from build123d import *

# Parameters (mm, degrees)
SKETCH1_W           = 135
SKETCH1_H           = 93
SKETCH1_R           = 3
BOSS_EXTRUDE1_DEPTH = 7
BOSS_EXTRUDE2_DEPTH = 39
FILLET1_R           = 10
SKETCH3_R           = 15
BOSS_EXTRUDE3_DEPTH = 22
SKETCH5_W           = 20
SKETCH5_H           = 8
BOSS_EXTRUDE4_DEPTH = 23
SKETCH6_R           = 4
CUT_EXTRUDE1_DEPTH  = 97.033848199
SKETCH7_R           = 12.5
BOSS_EXTRUDE5_DEPTH = 25


with BuildPart() as part:
    # Sketch1 → Boss-Extrude1 (new body)
    with BuildSketch(Plane.XY):
        Rectangle(SKETCH1_W, SKETCH1_H)
        with Locations((-55, 34)):
            Circle(SKETCH1_R, mode=Mode.SUBTRACT)
        with Locations((55, 34)):
            Circle(SKETCH1_R, mode=Mode.SUBTRACT)
        with Locations((55, -34)):
            Circle(SKETCH1_R, mode=Mode.SUBTRACT)
        with Locations((-55, -34)):
            Circle(SKETCH1_R, mode=Mode.SUBTRACT)
    extrude(amount=BOSS_EXTRUDE1_DEPTH)

    # Sketch2 → Boss-Extrude2 (add)
    with BuildSketch(Plane.XY.offset(7)):
        with BuildLine():
            Line((-36.5, 33), (36.5, 33))
            ThreePointArc((36.5, 33), (50.642135624, 27.142135624), (56.5, 13))
            Line((56.5, 13), (56.5, -13))
            ThreePointArc((56.5, -13), (50.642135624, -27.142135624), (36.5, -33))
            Line((36.5, -33), (-36.5, -33))
            ThreePointArc((-36.5, -33), (-50.642135624, -27.142135624), (-56.5, -13))
            Line((-56.5, -13), (-56.5, 13))
            ThreePointArc((-56.5, 13), (-50.642135624, 27.142135624), (-36.5, 33))
        make_face()
        with BuildLine():
            Line((-52.5, 13), (-52.5, -13))
            ThreePointArc((-52.5, -13), (-47.813708499, -24.313708499), (-36.5, -29))
            Line((-36.5, -29), (36.5, -29))
            ThreePointArc((36.5, -29), (47.813708499, -24.313708499), (52.5, -13))
            Line((52.5, -13), (52.5, 13))
            ThreePointArc((52.5, 13), (47.813708499, 24.313708499), (36.5, 29))
            Line((36.5, 29), (-36.5, 29))
            ThreePointArc((-36.5, 29), (-47.813708499, 24.313708499), (-52.5, 13))
        make_face(mode=Mode.SUBTRACT)
    extrude(amount=BOSS_EXTRUDE2_DEPTH)

    # Fillet1
    fillet1_edges = [part.edges().sort_by_distance(p)[0] for p in [
        (-67.5, -46.5, 3.5),
        (-67.5, 46.5, 3.5),
        (67.5, 46.5, 3.5),
        (67.5, -46.5, 3.5),
    ]]
    fillet(fillet1_edges, radius=FILLET1_R)

    # Sketch3 → Boss-Extrude3 (add)
    with BuildSketch(Plane(origin=(0, 0, 0), x_dir=(-1, 0, 0), z_dir=(0, 0, -1))):
        with Locations(Location((-35.5, 0, 0), (0, 0, 180))):
            Circle(SKETCH3_R)
        with Locations(Location((35.5, 0, 0), (0, 0, 180))):
            Circle(SKETCH3_R)
    extrude(amount=BOSS_EXTRUDE3_DEPTH)

    # Sketch5 → Boss-Extrude4 (add)
    with BuildSketch(Plane(origin=(0, 0, -22), x_dir=(-1, 0, 0), z_dir=(0, 0, -1))):
        with Locations((-35.5, 0)):
            Rectangle(SKETCH5_W, SKETCH5_H)
        with Locations((35.5, 0)):
            Rectangle(SKETCH5_W, SKETCH5_H)
    extrude(amount=BOSS_EXTRUDE4_DEPTH)

    # Sketch6 → Cut-Extrude1 (cut, through all)
    with BuildSketch(Plane(origin=(0, 4, 0), x_dir=(1, 0, 0), z_dir=(0, 1, 0))):
        with Locations(Location((35.5, 35, 0), (0, 0, 270))):
            Circle(SKETCH6_R)
        with Locations(Location((-35.5, 35, 0), (0, 0, 270))):
            Circle(SKETCH6_R)
    extrude(amount=-CUT_EXTRUDE1_DEPTH, mode=Mode.SUBTRACT)

    # Sketch7 → Boss-Extrude5 (add)
    with BuildSketch(Plane.XY.offset(7)):
        with Locations((-35.5, 0)):
            Circle(SKETCH7_R)
        with Locations((35.5, 0)):
            Circle(SKETCH7_R)
    extrude(amount=BOSS_EXTRUDE5_DEPTH)


solid = part.part
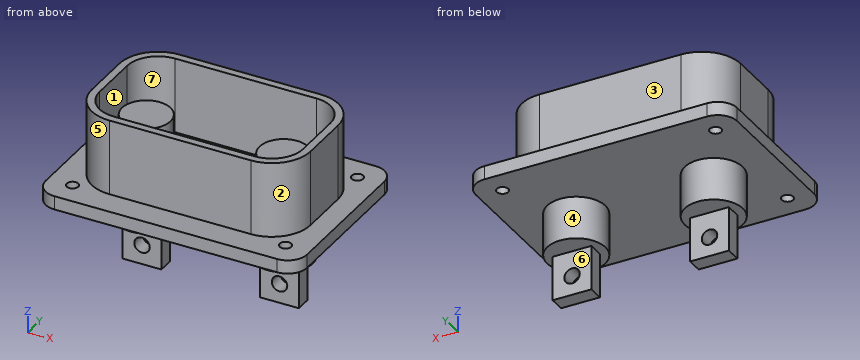
CAD build for the part. Positions are in the model's coordinates, mm. Face numbers are marked on the shaded views. A direction names the side the tool comes from. Round coordinates to 2 decimals unless told otherwise and drop trailing zeros. Write each loop counter-clockwise with the first axis right and the second up, starting at its lowest first coordinate (ties: lowest second). Pieces come first, ordered by that corner, then holes. Notation, with made-up numbers: (17.5, 13.5) -> (59.5, 13.5) arc R23 cw to (59.5, 37.5) -> close; hole circle Ø7 at (18.25, 13.25). An arc over 180 degrees is marked (long way). Answer as a JSON object with one key per item and string values.
(1) Band-saw the part on B-B, the plane x = 19. List the corners of the cut face in (y, z), then the cut area to 3 significant figures.
Reported:
{"outline": "(-46.5, 0) -> (46.5, 0) -> (46.5, 7) -> (33, 7) -> (33, 46) -> (29, 46) -> (29, 7) -> (-29, 7) -> (-29, 46) -> (-33, 46) -> (-33, 7) -> (-46.5, 7) -> close", "area": "963 mm^2"}
(2) Band-saw the part on C-C, the plane z = -35. List the corners of the cut face in (x, y).
Reported:
{"outline": "(-45.5, -4) -> (-39.5, -4) -> (-39.5, 4) -> (-45.5, 4) -> close; (-31.5, -4) -> (-25.5, -4) -> (-25.5, 4) -> (-31.5, 4) -> close; (25.5, -4) -> (31.5, -4) -> (31.5, 4) -> (25.5, 4) -> close; (39.5, -4) -> (45.5, -4) -> (45.5, 4) -> (39.5, 4) -> close"}
(3) Which spindle directions (+Z, -Z, +X, -X, +Y, -Y) get a long thin tool onto all of the face, cutting with end or side? Do the marked faces 4, 5, 6 and 7. Say none if no direction does.
Reported:
{"face 4": "-Z", "face 5": "+Z, -X, -Y", "face 6": "-Z, +X, -X, +Y", "face 7": "+Z"}
(4) Two-plate mould, pull along Y, no slides. Class the marked faces 1, 2 and 3: +Y half, -Y half, draft (parallel to the pull), parting line (faces both ways), or undercut.
Reported:
{"face 1": "undercut", "face 2": "-Y half", "face 3": "+Y half"}
(5) Probe probe 1 along Y at (x, z) = (55, 1); probe 2 along X at (y, z) = (1.75, -35); probe 3 along Y at (x, z) = (36, 19). List the from-to ranges inside material, lowest first. Write a range as [from, to].
Reported:
{"probe 1": "y = [-46.5, -37], [-31, 31], [37, 46.5]", "probe 2": "x = [-45.5, -39.5], [-31.5, -25.5], [25.5, 31.5], [39.5, 45.5]", "probe 3": "y = [-33, -29], [-12.49, 12.49], [29, 33]"}
(6) Band-saw the part on A-A, the plane z = 20. List the corners of the cut face in (x, y).
Reported:
{"outline": "(-56.5, -13) arc R20 ccw to (-36.5, -33) -> (36.5, -33) arc R20 ccw to (56.5, -13) -> (56.5, 13) arc R20 ccw to (36.5, 33) -> (-36.5, 33) arc R20 ccw to (-56.5, 13) -> close; circle Ø25 at (-35.5, 0); circle Ø25 at (35.5, 0); hole (-52.5, -13) arc R16 ccw to (-36.5, -29) -> (36.5, -29) arc R16 ccw to (52.5, -13) -> (52.5, 13) arc R16 ccw to (36.5, 29) -> (-36.5, 29) arc R16 ccw to (-52.5, 13) -> close"}
(7) Pin check, flat tips, straight feed: P1, Ø6.5, axis at y = -0.5, z = -34, coming from the -X side; P2, Ø8, axis at y = 5.5, z = 32, coming from the +X side; P3, Ø16, axis at x = 33.5, z = -36, coming from the -Y side. Stop position of each tip, or through.
Reported:
{"P1": "stops at x = -45.5", "P2": "stops at x = 56.5", "P3": "stops at y = -4"}
(8) Band-saw the part on D-D, the plane z = 2.5. List the corners of the cut face in (x, y).
Reported:
{"outline": "(-67.5, -36.5) arc R10 ccw to (-57.5, -46.5) -> (57.5, -46.5) arc R10 ccw to (67.5, -36.5) -> (67.5, 36.5) arc R10 ccw to (57.5, 46.5) -> (-57.5, 46.5) arc R10 ccw to (-67.5, 36.5) -> close; hole circle Ø6 at (-55, -34); hole circle Ø6 at (-55, 34); hole circle Ø6 at (55, -34); hole circle Ø6 at (55, 34)"}
